For this review, take the finished solid that the model builds, in its own axes (mm). A direction names the side the tool comes from. Give positions to 0.01 mm unless a question says otherwise; leave off trailing zeros. Write each loop counter-clockwise with the first axis right and the second up, starting at its lowest first coordinate (ties: lowest second). Pieces come first, ordered by that corner, then holes. Notation, with made-up numbers: M 13,-35.5 L 24,-35.5 A24 cw 24,-25.5 Z; hole C 3.25,17.5 d1. An arc over 180 degrees is marked long. Answer as a JSON object with one key per item and string values. Group by question number.
```python
from build123d import *

# Parameters (mm, degrees)
DODANIE_WYCI_GNI_CIE1_DEPTH = 46.5
WYTNIJ_WYCI_GNI_CIE1_DEPTH  = 2
SZKIC3_R                    = 3.25
WYTNIJ_WYCI_GNI_CIE2_DEPTH  = 2
DODANIE_WYCI_GNI_CIE2_DEPTH = 2
SZKIC5_W                    = 6.61
SZKIC5_H                    = 14.6
SZKIC5_W_2                  = 13.12
SZKIC5_H_2                  = 17.13
WYTNIJ_WYCI_GNI_CIE3_DEPTH  = 2
SKETCH1_R                   = 2
CUT_EXTRUDE1_DEPTH          = 5


with BuildPart() as part:
    # Szkic1 → Dodanie-wyci_gni_cie1 (new body)
    with BuildSketch(Plane.XY):
        with BuildLine():
            Line((-51.3, -64), (51.3, -64))
            ThreePointArc((51.3, -64), (59.785281374, -60.485281374), (63.3, -52))
            Line((63.3, -52), (63.3, 52))
            ThreePointArc((63.3, 52), (59.785281374, 60.485281374), (51.3, 64))
            Line((51.3, 64), (-51.3, 64))
            ThreePointArc((-51.3, 64), (-59.785281374, 60.485281374), (-63.3, 52))
            Line((-63.3, 52), (-63.3, -52))
            ThreePointArc((-63.3, -52), (-59.785281374, -60.485281374), (-51.3, -64))
        make_face()
    extrude(amount=DODANIE_WYCI_GNI_CIE1_DEPTH)

    # Szkic2 → Wytnij-wyci_gni_cie1 (cut)
    with BuildSketch(Plane(origin=(0, 64, 0), x_dir=(1, 0, 0), z_dir=(0, 1, 0))):
        with BuildLine():
            Line((-48.65, -31.2), (-48.65, -40.2))
            ThreePointArc((-48.65, -40.2), (-48.210660172, -41.260660172), (-47.15, -41.7))
            Line((-47.15, -41.7), (46.85, -41.7))
            ThreePointArc((46.85, -41.7), (47.910660172, -41.260660172), (48.35, -40.2))
            Line((48.35, -40.2), (48.35, -31.2))
            ThreePointArc((48.35, -31.2), (47.910660172, -30.139339828), (46.85, -29.7))
            Line((46.85, -29.7), (-47.15, -29.7))
            ThreePointArc((-47.15, -29.7), (-48.210660172, -30.139339828), (-48.65, -31.2))
        make_face()
    wytnij_wyci_gni_cie1 = extrude(amount=-WYTNIJ_WYCI_GNI_CIE1_DEPTH, mode=Mode.SUBTRACT)

    # Szkic3 → Wytnij-wyci_gni_cie2 (cut)
    with BuildSketch(Plane.ZY.offset(63.3)):
        with BuildLine():
            ThreePointArc((29.5, -45.8), (28.439339828, -45.360660172), (28, -44.3))
            Line((28, -44.3), (28, 43.7))
            ThreePointArc((28, 43.7), (28.439339828, 44.760660172), (29.5, 45.2))
            Line((29.5, 45.2), (38.5, 45.2))
            ThreePointArc((38.5, 45.2), (39.560660172, 44.760660172), (40, 43.7))
            Line((40, 43.7), (40, -44.3))
            ThreePointArc((40, -44.3), (39.560660172, -45.360660172), (38.5, -45.8))
            Line((38.5, -45.8), (29.5, -45.8))
        make_face()
        with BuildLine():
            Line((13.72769909, -23), (13.72769909, -28.8))
            ThreePointArc((13.72769909, -28.8), (15.37769909, -30.45), (17.02769909, -28.8))
            Line((17.02769909, -28.8), (17.02769909, -23))
            ThreePointArc((17.02769909, -23), (15.37769909, -21.35), (13.72769909, -23))
        make_face()
        with BuildLine():
            Line((13.72769909, -3.9), (13.72769909, -9.7))
            ThreePointArc((13.72769909, -9.7), (15.37769909, -11.35), (17.02769909, -9.7))
            Line((17.02769909, -9.7), (17.02769909, -3.9))
            ThreePointArc((17.02769909, -3.9), (15.37769909, -2.25), (13.72769909, -3.9))
        make_face()
        with Locations((15.37769909, 10.1)):
            Circle(SZKIC3_R)
    extrude(amount=-WYTNIJ_WYCI_GNI_CIE2_DEPTH, mode=Mode.SUBTRACT)

    # Szkic3_3 → Dodanie-wyci_gni_cie2 (add)
    with BuildSketch(Plane.ZY.offset(63.3)):
        with BuildLine():
            Line((12.37769909, 31.6), (12.37769909, 23.1))
            ThreePointArc((12.37769909, 23.1), (12.670592309, 22.392893219), (13.37769909, 22.1))
            Line((13.37769909, 22.1), (17.37769909, 22.1))
            ThreePointArc((17.37769909, 22.1), (18.084805871, 22.392893219), (18.37769909, 23.1))
            Line((18.37769909, 23.1), (18.37769909, 31.6))
            ThreePointArc((18.37769909, 31.6), (18.084805871, 32.307106781), (17.37769909, 32.6))
            Line((17.37769909, 32.6), (13.37769909, 32.6))
            ThreePointArc((13.37769909, 32.6), (12.670592309, 32.307106781), (12.37769909, 31.6))
        make_face()
    extrude(amount=DODANIE_WYCI_GNI_CIE2_DEPTH)

    # Lustro1: Wytnij-wyci_gni_cie1 across plane
    add(wytnij_wyci_gni_cie1.mirror(Plane.ZX), mode=Mode.SUBTRACT)

    # Szkic5 → Wytnij-wyci_gni_cie3 (cut)
    with BuildSketch(Plane(origin=(63.3, 0, 0), x_dir=(0, 0, -1), z_dir=(1, 0, 0))):
        with BuildLine():
            Line((-39.86, 49.36), (-32.58, 49.36))
            ThreePointArc((-32.58, 49.36), (-31.165786438, 48.774213562), (-30.58, 47.36))
            Line((-30.58, 47.36), (-30.58, -18.86))
            ThreePointArc((-30.58, -18.86), (-31.165786438, -20.274213562), (-32.58, -20.86))
            Line((-32.58, -20.86), (-39.86, -20.86))
            ThreePointArc((-39.86, -20.86), (-41.274213562, -20.274213562), (-41.86, -18.86))
            Line((-41.86, -18.86), (-41.86, 47.36))
            ThreePointArc((-41.86, 47.36), (-41.274213562, 48.774213562), (-39.86, 49.36))
        make_face()
        with BuildLine():
            Line((-21.12, -44.41), (-12.62, -44.41))
            ThreePointArc((-12.62, -44.41), (-11.912893219, -44.702893219), (-11.62, -45.41))
            Line((-11.62, -45.41), (-11.62, -48))
            ThreePointArc((-11.62, -48), (-11.912893219, -48.707106781), (-12.62, -49))
            Line((-12.62, -49), (-21.12, -49))
            ThreePointArc((-21.12, -49), (-21.827106781, -48.707106781), (-22.12, -48))
            Line((-22.12, -48), (-22.12, -45.41))
            ThreePointArc((-22.12, -45.41), (-21.827106781, -44.702893219), (-21.12, -44.41))
        make_face()
        with Locations((-8.705, -4.63)):
            Rectangle(SZKIC5_W, SZKIC5_H)
        with Locations((-15.36, -26.725)):
            Rectangle(SZKIC5_W_2, SZKIC5_H_2)
        with Locations((-17.905, -4.63)):
            Rectangle(SZKIC5_W, SZKIC5_H)
        Polygon((-20.57, 9.9), (-5.24, 9.9), (-5.24, 12.83), (-7.82, 15.06), (-17.99, 15.06), (-20.57, 12.83), align=None)
        Polygon((-7.82, 27.77), (-5.24, 25.54), (-5.24, 22.61), (-20.57, 22.61), (-20.57, 25.54), (-17.99, 27.77), align=None)
        with Locations((-17.905, 42.04)):
            Rectangle(SZKIC5_W, SZKIC5_H)
        with Locations((-8.705, 42.04)):
            Rectangle(SZKIC5_W, SZKIC5_H)
    extrude(amount=-WYTNIJ_WYCI_GNI_CIE3_DEPTH, mode=Mode.SUBTRACT)

    # Sketch1 → Cut-Extrude1 (cut)
    with BuildSketch(Plane(origin=(0, 0, 0), x_dir=(-1, 0, 0), z_dir=(0, 0, -1))):
        with Locations((-43, 0)):
            Circle(SKETCH1_R)
        with Locations((43, 0)):
            Circle(SKETCH1_R)
    extrude(amount=-CUT_EXTRUDE1_DEPTH, mode=Mode.SUBTRACT)


solid = part.part
```
Item 1: To check wall thickness, follow probe 1 along Y at (x, z) = (-43, 3.7); probe 2 along X at (y, z) = (-47.5, 15); probe 3 along X at (y, z) = (-35, 5). State the ranges of each line that lie inside material, in increasing order.
Item 2: Draft analysis for pull direction Z (two halves, no side actions). For faces 1 (the cylindrical face through (-41, 0, 2)), 2 (the flat face through (-43, 0, 5)), 3 (the cylindrical face through (-62.314, 11.076, 18.478)), state which applies: released by +Z, released by -Z, zero draft, split by the parting line, or undercut.
Item 3: Machinability: for faces 4 (the flat face through (-1, -62, 36)), 5 (the flat face through (-61.3, -26, 15)), 6 (the flat face through (-1, 62, 36)), 7 (the flat face through (61.3, -5, 18)), which of the approach directions +Z, -Z, +X, -X, +Y, -Y give a long, thin tool a straight path to every point of the face, cutting with its end or side? Answer none if there is none.
Item 4: Consider section D-D (y = -55.5). Give the boundary of the cut face in (x, z).
Item 5: Consider section B-B (y = 0). Give the boundary of the cut face in (x, z).
Item 6: Insertion check: P1, Ø1.6, axis at x = -62.5, z = 34.5, coming from the +Y side; P2, Ø1, axis at x = 62.5, z = 35.5, coming from the +Y side; P3, Ø1.5, axis at y = 42, z = 15, coming from the -X side. Each pin has a flat end and moves straight along its axis. Give the tip position at first contact, or say it passes through.
Item 7: Consider section C-C (y = -39). Give the boundary of the cut face in (x, z), plus the area to 3 significant figures.
Item 8: Consider section A-A (z = 35.5). Give the boundary of the cut face in (x, y).
Result set:
{
 "1": {"probe 1": "y = -64 to -2, 2 to 64", "probe 2": "x = -63.3 to 61.3", "probe 3": "x = -63.3 to 63.3"},
 "2": {"face 1": "zero draft", "face 2": "released by -Z", "face 3": "undercut"},
 "3": {"face 4": "-Y", "face 5": "-X", "face 6": "+Y", "face 7": "+X"},
 "4": {"outline": "M -62.78,0 L 62.78,0 L 62.78,46.5 L -62.78,46.5 Z"},
 "5": {"outline": "M -63.3,0 L -45,0 L -45,5 L -41,5 L -41,0 L 41,0 L 41,5 L 45,5 L 45,0 L 63.3,0 L 63.3,5.4 L 61.3,5.4 L 61.3,12.01 L 63.3,12.01 L 63.3,14.6 L 61.3,14.6 L 61.3,21.21 L 63.3,21.21 L 63.3,30.58 L 61.3,30.58 L 61.3,41.86 L 63.3,41.86 L 63.3,46.5 L -63.3,46.5 L -63.3,40 L -61.3,40 L -61.3,28 L -63.3,28 Z"},
 "6": {"P1": "stops at y = 57.99", "P2": "stops at y = 57.43", "P3": "stops at x = -63.3"},
 "7": {"outline": "M -63.3,0 L 63.3,0 L 63.3,46.5 L -63.3,46.5 L -63.3,40 L -61.3,40 L -61.3,28 L -63.3,28 Z", "area": "5,860 mm^2"},
 "8": {"outline": "M -63.3,-52 A12 ccw -51.3,-64 L -48.65,-64 L -48.65,-62 L 48.35,-62 L 48.35,-64 L 51.3,-64 A12 ccw 63.3,-52 L 63.3,-20.86 L 61.3,-20.86 L 61.3,49.36 L 63.3,49.36 L 63.3,52 A12 ccw 51.3,64 L 48.35,64 L 48.35,62 L -48.65,62 L -48.65,64 L -51.3,64 A12 ccw -63.3,52 L -63.3,45.2 L -61.3,45.2 L -61.3,-45.8 L -63.3,-45.8 Z"}
}
